Autodesk Inventor part; units mm, degrees
ref_plane "YZ Plane" through (0, 0, 0) normal (1, 0, 0) x (0, 1, 0)
ref_plane "XZ Plane" through (0, 0, 0) normal (0, 1, 0) x (-1, 0, 0)
ref_plane "XY Plane" through (0, 0, 0) normal (0, 0, 1) x (1, 0, 0)
sketch "Sketch1" plane through (0, 0, 0) normal (1, 0, 0) x (0, 1, 0)
  line L0 (0, 0) -> (125, 0)
  line L1 (125, 0) -> (125, -2)
  line L2 (125, -2) -> (0, -2)
  line L3 (0, -2) -> (0, 0)
  line L4 (125, 0) -> (123, 0)
  line L5 (123, 0) -> (123, -25)
  line L6 (123, -25) -> (125, -25)
  line L7 (125, -25) -> (125, 0)
  line L8 (0, 0) -> (2, 0)
  line L9 (2, 0) -> (2, -25)
  line L10 (2, -25) -> (0, -25)
  line L11 (0, -25) -> (0, 0)
  dimension "d0" = 125
  dimension "d1" = 2
  dimension "d2" = 2
  dimension "d3" = 25
  dimension "d4" = 2
  dimension "d5" = 25
extrude "Extrusion1" add sketch "Sketch1" along normal blind 100
sketch "Sketch2" plane through (0, 125, 0) normal (0, 1, 0) x (1, 0, 0)
  circle A0 centre (20, 12.5) radius 2.75
  circle A1 centre (50, 12.5) radius 2.75
  circle A2 centre (80, 12.5) radius 2.75
  line L0 (100, 25) -> (100, 0)
  line L1 (0, 25) -> (0, 0)
  line L2 (0, 25) -> (100, 25)
  dimension "d8" = 5.5
  dimension "d9" = 5.5
  dimension "d10" = 5.5
  dimension "d11" = 20
  dimension "d12" = 20
  dimension "d13" = 50
  dimension "d14" = 12.5
  dimension "d15" = 12.5
  dimension "d16" = 12.5
extrude "Extrusion2" cut sketch "Sketch2" against normal blind 125
properties part number "Vertical Plate Support" material "Aluminum 6061"
Input: part model. Units: mm. Frame: model coordinates. A direction names the side the tool comes from. Round coordinates to 2 decimals unless told otherwise and drop trailing zeros. Write each loop counter-clockwise with the first axis right and the second up, starting at its lowest first coordinate (ties: lowest second). Pieces come first, ordered by that corner, then holes.
1) Cut plane B-B (z = -6). Return the cut outline in (x, y), then the cut area to 3 significant figures.
2) Cut plane A-A (z = -12.5). Count the separate pieces of the cut face and the enclosed holes in it, then the cut area to 3 significant figures.
3) Cut plane D-D (x = 54.5). Return the cut outline in (y, z), then the cut area to 3 significant figures.
4) Ray query, L1, parallel to X at y = 1.5, z = -12.5; L2, parallel to Z at x = 20, y = 0.95; L3, parallel to Y at x = 30, z = -11. Return the intervals inside material, ascending.
5) Contact query for flat-ended pins moving along their axis: P1, Ø10, axis at y = 82.5, z = -11.5, coming from the -X side; P2, Ø8, axis at x = 45.5, y = 31.5, coming from the -Z side. Output: stop coordinate, or through.
6) Reachability of faces 1 (the flat face through (49.3, 125, -9.5)), 2 (the flat face through (49, 63, -2)) from +Z, -Z, +X, -X, +Y, -Y: full face, straight path, thin tool, end or side. Return the list, or none.
7) Draft query along Z for faces 3 (the flat face through (49, 2, -16)), 4 (the cylindrical face through (17.253, 124.014, -12.621)), 5 (the flat face through (49, 62, 0)), 6 (the cylindrical face through (17.253, 1.014, -12.621)). Return one class per face: pulls with the +Z half, pulls with the -Z half, needs draft (parallel to the pull), parting line crosses it, or undercut.
8) Cut plane C-C (x = 80). Return the cut outline in (y, z).
Geometry says:
1. outline: (0, 0) - (100, 0) - (100, 2) - (0, 2) - close; (0, 123) - (100, 123) - (100, 125) - (0, 125) - close
1. area: 400 mm2
2. separate pieces: 8
2. enclosed holes: 0
2. area: 334 mm2
3. outline: (0, -25) - (2, -25) - (2, -2) - (123, -2) - (123, -25) - (125, -25) - (125, 0) - (0, 0) - close
3. area: 342 mm2
4. L1: x = 0 to 17.25, 22.75 to 47.25, 52.75 to 77.25, 82.75 to 100
4. L2: z = -25 to -15.25, -9.75 to 0
4. L3: y = 0 to 2, 123 to 125
5. P1: passes through
5. P2: stops at z = -2
6. face 1: +Z, -Z, +X, -X, +Y
6. face 2: -Z, +X, -X
7. face 3: needs draft
7. face 4: undercut
7. face 5: pulls with the +Z half
7. face 6: undercut
8. outline: (0, -25) - (2, -25) - (2, -15.25) - (0, -15.25) - close; (0, -9.75) - (2, -9.75) - (2, -2) - (123, -2) - (123, -9.75) - (125, -9.75) - (125, 0) - (0, 0) - close; (123, -25) - (125, -25) - (125, -15.25) - (123, -15.25) - close
